```python
from build123d import *

# Parameters (mm, degrees)
CHAMFER1_SIZE = 1.5875
CHAMFER2_SIZE = 1.5875


with BuildPart() as part:
    # Sketch1 → Revolve1 (revolve)
    with BuildSketch(Plane.XY):
        Polygon((0, 0), (0, 9.525), (10.7188, 9.525), (10.7188, 12.7), (65.4812, 12.7), (65.4812, 9.525), (76.2, 9.525), (76.2, 0), align=None)
    revolve(axis=Axis((76.2, 0, 0), (-1, 0, 0)))

    # Chamfer1
    chamfer1_edges = [part.edges().sort_by_distance(p)[0] for p in [
        (76.2, -9.525, 0),
    ]]
    chamfer(chamfer1_edges, length=CHAMFER1_SIZE)

    # Chamfer2
    chamfer2_edges = [part.edges().sort_by_distance(p)[0] for p in [
        (0, -9.525, 0),
    ]]
    chamfer(chamfer2_edges, length=CHAMFER2_SIZE)


solid = part.part
```
Geometry: final body of the model. Coordinates: model frame, mm. A direction names the side the tool comes from. Give positions to 0.01 mm unless a question says otherwise; leave off trailing zeros. Loops run counter-clockwise (first coordinate to the right, second up) from the corner with the lowest first, then second, coordinate; pieces in that order, holes last. Notation, with made-up numbers: (82, -0.5) -> (87, -0.5) arc R28 cw to (87, 26.5) -> close; hole circle Ø3 at (30.25, 17.25). An arc over 180 degrees is marked (long way). Return JSON: item names as keys, results as strings.
Item 1: Section A-A, the plane z = 0. Output: boundary loops of the cut face in (x, y) (1 decimal), plus the area to 3 significant figures.
Filled in:
{"outline": "(0, -7.9) -> (1.6, -9.5) -> (10.7, -9.5) -> (10.7, -12.7) -> (65.5, -12.7) -> (65.5, -9.5) -> (74.6, -9.5) -> (76.2, -7.9) -> (76.2, 7.9) -> (74.6, 9.5) -> (65.5, 9.5) -> (65.5, 12.7) -> (10.7, 12.7) -> (10.7, 9.5) -> (1.6, 9.5) -> (0, 7.9) -> close", "area": "1,790 mm^2"}
Item 2: Section C-C, the plane x = 68.5. Output: boundary loops of the cut face in (y, z) (3 decimals).
Filled in:
{"outline": "circle Ø19.05 at (0, 0)"}
Item 3: Access query for faces 1 (the flat face through (10.719, -5, -9)), 2 (the flat face through (65.481, 5, -9)), 3 (the flat face through (0, 0, 0)). Directions: +Z, -Z, +X, -X, +Y, -Y. A direction counts if a zero-diameter tool reaches every point of the face in a straight line with its end or side. Return the directions, or none.
Filled in:
{"face 1": "-X", "face 2": "+X", "face 3": "+Z, -Z, -X, +Y, -Y"}
Item 4: Section D-D, the plane x = 58. Output: boundary loops of the cut face in (y, z).
Filled in:
{"outline": "circle Ø25.4 at (0, 0)"}
Item 5: Line query: line 1 (X direction, y = -0.75, z = -9.75); line 2 (Z direction, x = 64, y = 0.5); line 3 (Z direction, x = 4, y = -0.25). Output: solid intervals per line, ascending.
Filled in:
{"line 1": "10.72 to 65.48", "line 2": "-12.69 to 12.69", "line 3": "-9.52 to 9.52"}
Item 6: Pin query (flat end, axial travel): P1, Ø2, axis at x = 57, y = -3.5, coming from the -Z side; P2, Ø1.5, axis at x = 32.5, y = -5.5, coming from the +Z side; P3, Ø3, axis at x = 47.5, y = 10, coming from the +Z side. Return the tip coordinate at first contact, or that it passes through.
Filled in:
{"P1": "z = -12.45", "P2": "z = 11.78", "P3": "z = 9.44"}
